Autodesk Inventor part; units mm, degrees
ref_plane "YZ Plane" through (0, 0, 0) normal (1, 0, 0) x (0, 1, 0)
ref_plane "XZ Plane" through (0, 0, 0) normal (0, 1, 0) x (-1, 0, 0)
ref_plane "XY Plane" through (0, 0, 0) normal (0, 0, 1) x (1, 0, 0)
sketch "Sketch1" plane through (0, 0, 0) normal (0, 0, 1) x (1, 0, 0)
  line L0 (-85, -9) -> (85, -9)
  line L1 (85, -9) -> (85, 9)
  line L2 (85, 9) -> (-85, 9)
  line L3 (-85, 9) -> (-85, -9)
  line L4 (-85, -9) -> (85, 9) construction
  line L5 (85, -9) -> (-85, 9) construction
  point P0 (0, 0)
  dimension "d3" = 18
  dimension "d26" = 170
extrude "Extrusion1" add sketch "Sketch1" along normal mid plane 4
sketch "Sketch2" plane through (0, 0, -2) normal (0, 0, -1) x (-1, 0, 0)
  line L0 (0, -15) -> (0, 15) construction
  line L1 (85, 9) -> (-85, 9)
  circle A0 centre (73, -4) radius 2.5
  arc A1 (73, 5.3986) -> (73, 1.6013) centre (73, 3.5) ccw
  line L2 (73, 3.5) -> (73, -4) construction
  line L3 (73, -4) -> (78.3033, -4) construction
  circle A2 centre (73, -4) radius 7.5 construction
  arc A3 (76.9608, -0.0392) -> (79.6458, 2.6458) centre (78.3033, 1.3033) ccw
  arc A4 (79.6458, 2.6458) -> (73, 5.3986) centre (73, -4) ccw
  arc A5 (76.9608, -0.0392) -> (73, 1.6013) centre (73, -4) ccw
  line L4 (85, -10.7625) -> (85, 10.7625) construction
  line L5 (73, -4) -> (78.3033, 1.3033) construction
  line L6 (78.3033, 1.3033) -> (78.3033, -4) construction
  line L7 (85, -9) -> (85, 9)
  line L8 (-85, -9) -> (85, -9)
  line L9 (-73, 3.5) -> (-73, -4) construction
  arc A6 (-73, 1.6013) -> (-73, 5.3986) centre (-73, 3.5) ccw
  circle A7 centre (-73, -4) radius 2.5
  arc A8 (-73, 1.6013) -> (-76.9608, -0.0392) centre (-73, -4) ccw
  line L10 (-73, -4) -> (-78.3033, -4) construction
  line L11 (-73, -4) -> (-78.3033, 1.3033) construction
  line L12 (-78.3033, 1.3033) -> (-78.3033, -4) construction
  circle A9 centre (-73, -4) radius 7.5 construction
  arc A10 (-73, 5.3986) -> (-79.6458, 2.6458) centre (-73, -4) ccw
  arc A11 (-79.6458, 2.6458) -> (-76.9608, -0.0392) centre (-78.3033, 1.3033) ccw
  line L13 (-85, -10.7625) -> (-85, 10.7625) construction
  line L14 (-85, -9) -> (-85, 9)
  point P0 (0, 0)
  point P1 (85, 0)
  point P2 (-85, 0)
  dimension "d40" = 5
  dimension "d41" = 3.7973
  dimension "d42" = 3.7973
  dimension "d43" = 15
  dimension "d44" = 12
  dimension "d45" = 5
extrude "Extrusion2" cut sketch "Sketch2" against normal through all contours A0 | A4 A3 A5 A1 | A8 A11 A10 A6 | A7
fillet "Fillet1" radius 2 4 edges at (-85, 9, 0) (-85, -9, 0) (85, 9, 0) (85, -9, 0)
sketch "Sketch5" plane through (0, 0, 2) normal (0, 0, 1) x (1, 0, 0)
  line L0 (0, -9) -> (0, 0) construction
  line L1 (0, 0) -> (0, 9) construction
  line L2 (83, 9) -> (-83, 9) construction
  line L3 (-83, -9) -> (83, -9) construction
  point P0 (0, -4.5)
  point P1 (0, 4.5)
hole "Hole2" at (0, -4.5, 2) at (0, 4.5, 2) direction (0, 0, -1) diameter 4.496 end through all
equation "\"d42\" = d41"
properties part number "CameraBase"
Work out the finished part from the listing and answer in its coordinate system (mm). A direction names the side the tool comes from. Give positions to 0.01 mm unless a question says otherwise; leave off trailing zeros. Write each loop counter-clockwise with the first axis right and the second up, starting at its lowest first coordinate (ties: lowest second). Pieces come first, ordered by that corner, then holes.
Q1. Straight lines are drawn through the part: L1, parallel to Y at x = 0, z = -1; L2, parallel to Y at x = -73, z = 0.3; L3, parallel to X at y = 4, z = 1.45. For each, find the intervals that lie inside material, in ascending order.
Answer:
L1: y = -9 to -6.75, -2.25 to 2.25, 6.75 to 9
L2: y = -9 to -6.5, -1.5 to 1.6, 5.4 to 9
L3: x = -85 to -77.93, -71.17 to -2.19, 2.19 to 71.17, 77.93 to 85
Q2. The part is cut by section A-A on x = 0. Give the vertices of the cut face in (y, z).
Answer:
outline: (-9, -2) - (-6.75, -2) - (-6.75, 2) - (-9, 2) - close; (-2.25, -2) - (2.25, -2) - (2.25, 2) - (-2.25, 2) - close; (6.75, -2) - (9, -2) - (9, 2) - (6.75, 2) - close
Q3. The part is cut by section B-B on z = 0. Give the vertices of the cut face in (x, y).
Answer:
outline: (-85, -7) arc R2 ccw to (-83, -9) - (83, -9) arc R2 ccw to (85, -7) - (85, 7) arc R2 ccw to (83, 9) - (-83, 9) arc R2 ccw to (-85, 7) - close; hole (-79.65, 2.65) arc R1.9 ccw to (-76.96, -0.04) arc R5.6 cw to (-73, 1.6) arc R1.9 ccw to (-73, 5.4) arc R9.4 ccw to start; hole circle Ø5 at (-73, -4); hole circle Ø4.5 at (0, -4.5); hole circle Ø4.5 at (0, 4.5); hole circle Ø5 at (73, -4); hole (73, 1.6) arc R5.6 cw to (76.96, -0.04) arc R1.9 ccw to (79.65, 2.65) arc R9.4 ccw to (73, 5.4) arc R1.9 ccw to start
Q4. For a pull along X with two mould halves and no side action, classify faces 3 (the face through (-76.644, 4.663, -0.028)), 4 (the face through (-85, 0, 0)), 5 (the face through (-1, 0, 2)) as released by +X, released by -X, zero draft, split by the parting line, or undercut.
Answer:
face 3: undercut
face 4: released by -X
face 5: zero draft
Q5. A tool of negligible diameter and unlimited length cuts with its end or side. For faces 1 (the face through (71.1, 3.5, 0)), 2 (the face through (85, 0, 0)), from which of +Z, -Z, +X, -X, +Y, -Y can it reach the whole face along a straight path? Write none if from no direction.
Answer:
face 1: +Z, -Z
face 2: +Z, -Z, +X, +Y, -Y
Q6. Given pin 1 (2.5 mm diameter, centred on x = 0, y = -4.5, fed in from -Z), flat-ended and moving along its own axis, determine where the tip first touches the part or whether it passes through.
Answer:
pin 1: passes through
Q7. The part is cut by section C-C on y = -4. Give the vertices of the cut face in (x, z), and give its area (3 significant figures).
Answer:
outline: (-85, -2) - (-75.5, -2) - (-75.5, 2) - (-85, 2) - close; (-70.5, -2) - (-2.19, -2) - (-2.19, 2) - (-70.5, 2) - close; (2.19, -2) - (70.5, -2) - (70.5, 2) - (2.19, 2) - close; (75.5, -2) - (85, -2) - (85, 2) - (75.5, 2) - close
area: 622 mm2
